Geometry: see drawing. Coordinates: mm, zero at the bounding-box minimum. A direction names the side the tool comes from. Coordinates: 2 decimals unless noted, no trailing zeros. Loops run counter-clockwise (first coordinate to the right, second up) from the corner with the lowest first, then second, coordinate; pieces in that order, holes last.
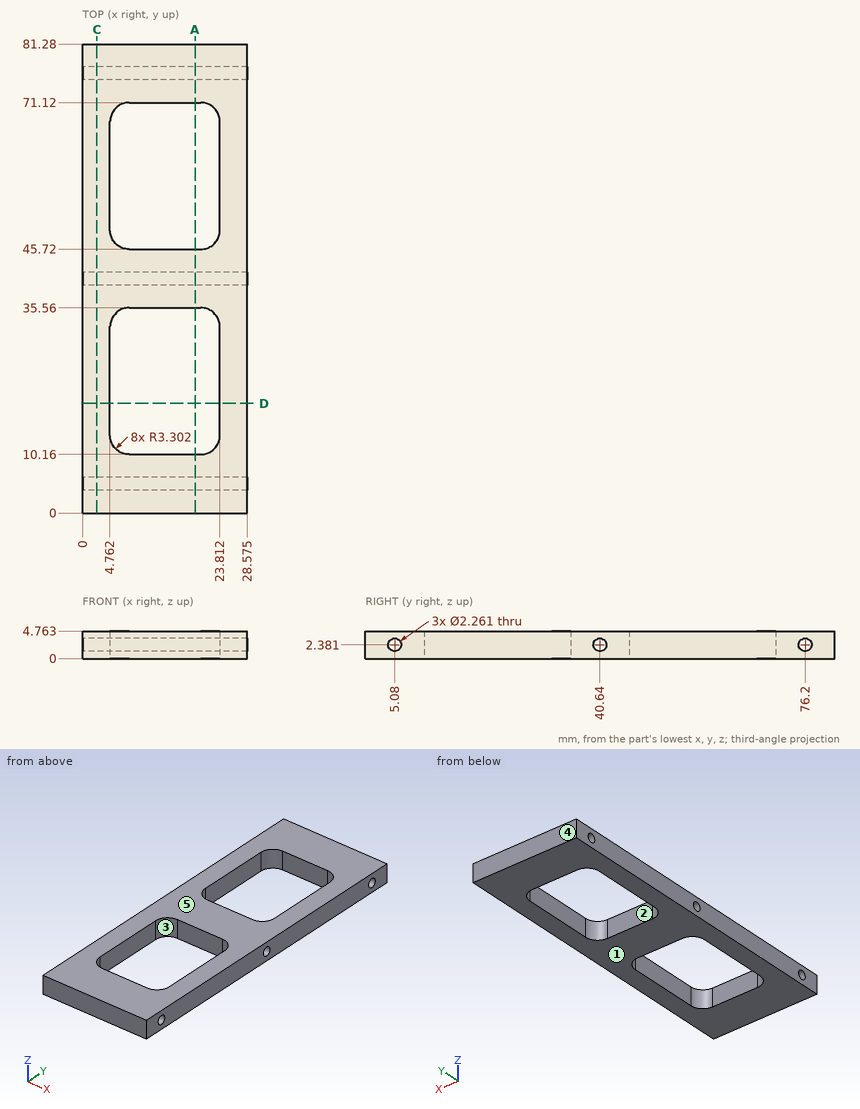
Item 1: Line query: L1, parallel to Y at x = 13.25, z = 0.6; L2, parallel to Y at x = 19.25, z = 2.3; L3, parallel to Z at x = 19.5, y = 76.2. Output: solid intervals per line, ascending.
Result:
L1: y = 0 to 10.16, 35.56 to 45.72, 71.12 to 81.28
L2: y = 0 to 3.95, 6.21 to 10.16, 35.56 to 39.51, 41.77 to 45.72, 71.12 to 75.07, 77.33 to 81.28
L3: z = 0 to 1.25, 3.51 to 4.76
Item 2: Reachability of the marked faces 1 and 2 from +Z, -Z, +X, -X, +Y, -Y: full face, straight path, thin tool, end or side. Return the list, or none.
Result:
face 1: -Z, +X, -X, +Y, -Y
face 2: +Z, -Z
Item 3: Mould query, pull axis Y, two halves, no side actions, for the marked faces 3, 4 and 5. Classes: +Y half, -Y half, draft (parallel to the pull), parting line (faces both ways), or undercut.
Result:
face 3: undercut
face 4: +Y half
face 5: draft
Item 4: Contact query for flat-ended pins moving along their axis: P1, Ø1.5, axis at x = 9, z = 1.5, coming from the -Y side; P2, Ø1.4, axis at y = 5.08, z = 2.38, coming from the -X side. Output: stop coordinate, or through.
Result:
P1: stops at y = 0
P2: passes through
Item 5: Section query C-C (x = 2.5). Output: boundary loops of the cut face in (y, z), then the cut area to 3 significant figures.
Result:
outline: (0, 0) - (81.28, 0) - (81.28, 4.76) - (0, 4.76) - close; hole circle Ø2.26 at (5.08, 2.38); hole circle Ø2.26 at (40.64, 2.38); hole circle Ø2.26 at (76.2, 2.38)
area: 375 mm2
Item 6: Section query A-A (x = 19.5). Output: boundary loops of the cut face in (y, z), then the cut area to 3 significant figures.
Result:
outline: (0, 0) - (10.16, 0) - (10.16, 4.76) - (0, 4.76) - close; (35.56, 0) - (45.72, 0) - (45.72, 4.76) - (35.56, 4.76) - close; (71.12, 0) - (81.28, 0) - (81.28, 4.76) - (71.12, 4.76) - close; hole circle Ø2.26 at (5.08, 2.38); hole circle Ø2.26 at (40.64, 2.38); hole circle Ø2.26 at (76.2, 2.38)
area: 133 mm2
Item 7: Section query D-D (y = 19). Output: boundary loops of the cut face in (x, z) (1 decimal).
Result:
outline: (0, 0) - (4.8, 0) - (4.8, 4.8) - (0, 4.8) - close; (23.8, 0) - (28.6, 0) - (28.6, 4.8) - (23.8, 4.8) - close
